Autodesk Inventor part; units mm, degrees
ref_plane "Work Plane1" through (0, 0, 5.08) normal (0, 0, 1) x (1, 0, 0)
ref_plane "Work Plane2" through (0, 0, 7.62) normal (0, 0, 1) x (1, 0, 0)
ref_plane "YZ Plane" through (0, 0, 0) normal (1, 0, 0) x (0, 1, 0)
sketch "Sketch1" plane through (0, 0, 0) normal (0, 0, 1) x (1, 0, 0)
  line L0 (0, 0) -> (27.94, 0)
  line L1 (27.94, 0) -> (27.94, 16.256)
  line L2 (27.94, 16.256) -> (0, 16.256)
  line L3 (0, 16.256) -> (0, 0)
  dimension "d0" = 27.94
  dimension "d1" = 16.256
extrude "Extrusion1" add sketch "Sketch1" along normal blind 10.16
fillet "Fillet1" radius 1.27 4 edges at (0, 16.256, 5.08) (27.94, 16.256, 5.08) (27.94, 0, 5.08) (0, 0, 5.08)
sketch "Sketch3" plane through (0, 0, 10.16) normal (0, 0, 1) x (1, 0, 0)
  arc A0 (0, 1.27) -> (1.27, 0) centre (1.27, 1.27) ccw
  line L0 (1.27, 0) -> (26.67, 0)
  arc A1 (26.67, 0) -> (27.94, 1.27) centre (26.67, 1.27) ccw
  line L1 (27.94, 1.27) -> (27.94, 14.986)
  arc A2 (27.94, 14.986) -> (26.67, 16.256) centre (26.67, 14.986) ccw
  line L2 (26.67, 16.256) -> (1.27, 16.256)
  arc A3 (1.27, 16.256) -> (0, 14.986) centre (1.27, 14.986) ccw
  line L3 (0, 14.986) -> (0, 1.27)
  line L4 (26.67, 16.256) -> (1.27, 16.256)
  line L5 (24.765, 16.256) -> (24.765, 18.542)
  line L6 (24.765, 18.542) -> (22.733, 18.542)
  line L7 (22.733, 18.542) -> (22.733, 16.256)
  point P0 (0, 0)
  dimension "d12" = 2.286
  dimension "d13" = 2.032
  dimension "d14" = 3.175
ref_plane "Work Plane1" through (0, 0, 5.08) normal (0, 0, 1) x (1, 0, 0)
sketch "Sketch4" plane through (0, 0, 5.08) normal (0, 0, 1) x (1, 0, 0)
  line L0 (24.765, 18.542) -> (22.733, 18.542)
  line L1 (22.733, 18.542) -> (22.733, 16.256)
  line L2 (24.765, 16.256) -> (24.765, 18.542)
  line L3 (22.733, 16.256) -> (24.765, 16.256)
  line L4 (26.67, 16.256) -> (1.27, 16.256)
  point P0 (0, 0)
extrude "Extrusion3" add sketch "Sketch4" along normal mid plane 2.032
fillet "Fillet2" radius 0.254 2 edges at (24.765, 18.542, 5.08) (22.733, 18.542, 5.08)
ref_plane "Work Plane2" through (0, 0, 7.62) normal (0, 0, 1) x (1, 0, 0)
sketch "Sketch5" plane through (0, 0, 7.62) normal (0, 0, 1) x (1, 0, 0)
  arc A0 (0, 1.27) -> (1.27, 0) centre (1.27, 1.27) ccw
  line L0 (1.27, 0) -> (26.67, 0)
  arc A1 (26.67, 0) -> (27.94, 1.27) centre (26.67, 1.27) ccw
  line L1 (27.94, 1.27) -> (27.94, 14.986)
  arc A2 (27.94, 14.986) -> (26.67, 16.256) centre (26.67, 14.986) ccw
  line L2 (26.67, 16.256) -> (1.27, 16.256)
  arc A3 (1.27, 16.256) -> (0, 14.986) centre (1.27, 14.986) ccw
  line L3 (0, 14.986) -> (0, 1.27)
  line L4 (0, 14.986) -> (0, 1.27)
  line L5 (0, 10.1931) -> (-10.16, 10.1931)
  line L6 (-10.16, 10.1931) -> (-10.16, 9.5581)
  line L7 (-10.16, 9.5581) -> (0, 9.5581)
  line L8 (0, 9.5581) -> (0, 10.1931)
  line L9 (0, 4.6288) -> (-10.16, 4.6288)
  line L10 (-10.16, 4.6288) -> (-10.16, 3.9938)
  line L11 (-10.16, 3.9938) -> (0, 3.9938)
  line L12 (0, 3.9938) -> (0, 4.6288)
  line L13 (11.4462, 0) -> (10.8112, 0)
  line L14 (10.8112, 0) -> (10.8112, -2.1198)
  line L15 (10.8112, -2.1198) -> (11.4462, -2.1198)
  line L16 (11.4462, -2.1198) -> (11.4462, 0)
  line L17 (10.8112, -2.1198) -> (1.7523, -4.475)
  line L18 (1.7523, -4.475) -> (1.912, -5.0896)
  line L19 (1.912, -5.0896) -> (11.4462, -2.6109)
  line L20 (11.4462, -2.6109) -> (11.4462, -2.1198)
  point P0 (0, 0)
  dimension "d19" = 10.16
  dimension "d20" = 0.635
  dimension "d21" = 0.635
  dimension "d22" = 0.635
extrude "Extrusion4" add sketch "Sketch5" against normal blind 5.08 contours L11 L10 L9 L3 | L0 L16 L15 L14 | L15 L20 L19 L18 L17 | L7 L6 L5 L3
fillet "Fillet3" radius 1.27 6 edges at (-10.16, 4.3113, 7.62) (-10.16, 9.8756, 7.62) (-10.16, 4.3113, 2.54) (-10.16, 9.8756, 2.54) (1.8322, -4.7823, 7.62) (1.8322, -4.7823, 2.54)
properties part number "LIMIT SWITCH"
CAD build for the part. Positions are in the model's coordinates, mm. A direction names the side the tool comes from. Give positions to 0.01 mm unless a question says otherwise; leave off trailing zeros. Order: outer loops, then holes, each group sorted by start corner. A loop starts at its lowest first (then second) coordinate and runs counter-clockwise, first axis right, second up. Notation, with made-up numbers: (37, -24.75) - (69, -24.75) arc R25 ccw to (69, -0.75) - close; hole circle Ø3 at (82, 48). An arc over 180 degrees is marked (long way). Write each question's results on one line, items separated by ' | '.
1. Saw through at D-D on x = 7. List the corners of the cut face in (y, z).
Calculated:
outline: (-3.77, 2.54) - (-3.11, 2.54) - (-3.11, 7.62) - (-3.77, 7.62) - close; (0, 0) - (16.26, 0) - (16.26, 10.16) - (0, 10.16) - close
2. Saw through at B-B on z = 1.75. List the corners of the cut face in (x, y), and give its area (3 significant figures).
Calculated:
outline: (0, 1.27) arc R1.27 ccw to (1.27, 0) - (26.67, 0) arc R1.27 ccw to (27.94, 1.27) - (27.94, 14.99) arc R1.27 ccw to (26.67, 16.26) - (1.27, 16.26) arc R1.27 ccw to (0, 14.99) - close | area: 453 mm2
3. Probe L1, parallel to Y at x = -7.5, z = 7; L2, parallel to X at y = 5.75, z = 2.25; L3, parallel to X at y = -2, z = 7.5. List the from-to ranges inside material, lowest first. Write a range as from..to.
Calculated:
L1: y = 3.99..4.63, 9.56..10.19 | L2: x = 0..27.94 | L3: x = 10.81..11.45
4. 3-axis set-ups, long thin cutter, end or side, ignore diameter. For faces 1 (the face through (7.8, -3.1, 2.54)), 2 (the face through (24, 17, 6.096)), 3 (the face through (24, 17, 4.064)), 4 (the face through (-5, 9.558, 5)): which of +Z, -Z, +X, -X, +Y, -Y reach the whole face in a straight line?
Calculated:
face 1: -Z, +X, -X, -Y | face 2: +Z, +X, -X, +Y | face 3: -Z, +X, -X, +Y | face 4: +Z, -Z, -X
5. Saw through at A-A on x = -8. List the corners of the cut face in (y, z).
Calculated:
outline: (3.99, 2.54) - (4.63, 2.54) - (4.63, 7.62) - (3.99, 7.62) - close; (9.56, 2.54) - (10.19, 2.54) - (10.19, 7.62) - (9.56, 7.62) - close
6. Pin check, flat tips, straight feed: pin 1 (2 mm diameter, centred on x = 14, z = 4, fed in from +Y); pin 2 (0.7 mm diameter, centred on x = -2.5, y = 10, fed in from -Z); pin 3 (2.5 mm diameter, centred on x = -5.5, z = 5.5, fed in from +Y). Stop position of each tip, or through.
Calculated:
pin 1: stops at y = 16.26 | pin 2: stops at z = 2.54 | pin 3: stops at y = 10.19
7. Saw through at C-C on x = 20. List the corners of the cut face in (y, z).
Calculated:
outline: (0, 0) - (16.26, 0) - (16.26, 10.16) - (0, 10.16) - close
